from build123d import *

# Parameters (mm, degrees)
F0_W             = 20
F0_H             = 20
F1_DEPTH         = 448
F2_R             = 2.1
F3_DEPTH         = 448.001
F4_R             = 1
F6_DEPTH         = 448.001
F6_COPIES3_COUNT = 2
F6_COPIES3_ANGLE = 90
F6_COPIES4_COUNT = 2
F6_COPIES4_ANGLE = 270
F6_COPIES6_COUNT = 2
F9_W             = 16.4
F9_H             = 6.8613203436
F10_DEPTH        = 448.001
F12_DEPTH        = 448


# Not quite as in the source:
# - a pattern or mirror of a feature is missing from the dataset's text; its kind, count and spacing are read off the source's solid


with BuildPart() as f1:
    # F0 (on Front) → F1 (new body)
    with BuildSketch(Plane.XZ):
        Rectangle(F0_W, F0_H)
    extrude(amount=F1_DEPTH)

    # F2 (on face) → F3 (cut, through all)
    with BuildSketch(Plane.XZ.offset(448)):
        Circle(F2_R)
    extrude(amount=-F3_DEPTH, mode=Mode.SUBTRACT)

    # F4
    f4_edges = [f1.edges().sort_by_distance(p)[0] for p in [
        (-10, -224, 10),
        (10, -224, 10),
    ]]
    fillet(f4_edges, radius=F4_R)

    # F5 (on face) → F6 (cut, through all)
    with BuildSketch(Plane.XZ.offset(448)):
        Polygon((0, 3.9006601718), (0, 10), (-2.84, 10), (-4.64, 10), (-2.84, 8.2), (-5.4993398282, 8.2), (-5.4993398282, 6.56), (-2.84, 3.9006601718), align=None)
        Polygon((-6.5693398282, 8.2), (-8.2, 8.2), (-7.0953059148, 7.0953059148), (-6.5693398282, 7.6212720014), align=None)
    f6 = extrude(amount=-F6_DEPTH, mode=Mode.SUBTRACT)

    # F6_copies: F6 across plane
    add(f6.mirror(Plane(origin=(0, 0, 0), x_dir=(-0.7071067812, 0, -0.7071067812), z_dir=(0.7071067812, 0, -0.7071067812))), mode=Mode.SUBTRACT)

    # F6_copies1: F6 across plane
    add(f6.mirror(Plane(origin=(0, 0, 0), x_dir=(0.7071067812, 0, -0.7071067812), z_dir=(-0.7071067812, 0, -0.7071067812))), mode=Mode.SUBTRACT)

    # F6_copies2: F6 across plane
    add(f6.mirror(Plane(origin=(0, 0, 0), x_dir=(0, 0, 1), z_dir=(1, 0, 0))), mode=Mode.SUBTRACT)

    # F6_copies3: F6 ×2 about axis
    f6_copies3_axis = Axis((0, 0, 0), (0, 1, 0))
    for i in range(1, F6_COPIES3_COUNT):
        add(f6.rotate(f6_copies3_axis, i * F6_COPIES3_ANGLE / (F6_COPIES3_COUNT - 1)), mode=Mode.SUBTRACT)

    # F6_copies4: F6 ×2 about axis
    f6_copies4_axis = Axis((0, 0, 0), (0, 1, 0))
    for i in range(1, F6_COPIES4_COUNT):
        add(f6.rotate(f6_copies4_axis, i * F6_COPIES4_ANGLE / (F6_COPIES4_COUNT - 1)), mode=Mode.SUBTRACT)

    # F6_copies5: F6 across plane
    add(f6.mirror(Plane(origin=(0, 0, 0), x_dir=(-1, 0, 0), z_dir=(0, 0, -1))), mode=Mode.SUBTRACT)

    # F6_copies6: F6 ×2 about axis
    f6_copies6_axis = Axis((0, 0, 0), (0, 1, 0))
    for i in range(1, F6_COPIES6_COUNT):
        add(f6.rotate(f6_copies6_axis, i * 360 / F6_COPIES6_COUNT), mode=Mode.SUBTRACT)

    # F8: F1 across face


with BuildPart() as f1_1:
    add(f1.part)
    add(f1.part.mirror(Plane(origin=(-7.32, -224, -10), x_dir=(1, 0, 0), z_dir=(0, 0, -1))))

    # F9 (on face) → F10 (cut, through all)
    with BuildSketch(Plane.XZ.offset(448)):
        with Locations((0, -10)):
            Rectangle(F9_W, F9_H)
    extrude(amount=-F10_DEPTH, mode=Mode.SUBTRACT)

    # F11 (on face) → F12 (join, through all)
    with BuildSketch(Plane.XZ.offset(448)):
        with BuildLine():
            ThreePointArc((-9, -10), (-9.7071067812, -9.7071067812), (-10, -9))
            Line((-10, -9), (-10, -11))
            ThreePointArc((-10, -11), (-9.7071067812, -10.2928932188), (-9, -10))
        make_face()
        with BuildLine():
            ThreePointArc((10, -9), (9.7071067812, -9.7071067812), (9, -10))
            ThreePointArc((9, -10), (9.7071067812, -10.2928932188), (10, -11))
            Line((10, -11), (10, -9))
        make_face()
        Polygon((5.9386796564, -6.9993398282), (8.2, -6.9993398282), (8.2, -6.5693398282), (5.5086796564, -6.5693398282), align=None)
        Polygon((-8.2, -6.5693398282), (-8.2, -6.9993398282), (-5.9386796564, -6.9993398282), (-5.5086796564, -6.5693398282), align=None)
    extrude(amount=-F12_DEPTH)


solid = f1_1.part
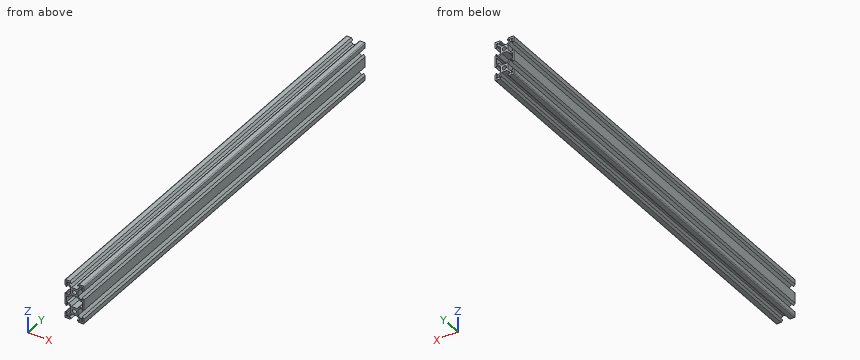
The model under review builds one solid part; all positions refer to its coordinate system, in mm. Give positions to 0.01 mm unless a question says otherwise; leave off trailing zeros. One line per question, with ' | ' between items. Start each with the question number.
Item 1: Wall thickness on line 1 (Z direction, x = 0, y = -333.5); line 2 (Z direction, x = 8, y = -54.5); line 3 (X direction, y = -407.5, z = 7): over which ranges is each line inside the solid? List them lowest first. Write a range as from..to.
Item 2: For pin 1 (3 mm diameter, centred on x = -4.5, y = -162, fed in from -Z); pin 2 (4 mm diameter, centred on y = -292, z = -22.5, fed in from +X); pin 3 (1.5 mm diameter, centred on y = -399.5, z = 3.5, fed in from +X); pin 4 (4.5 mm diameter, centred on x = -1, y = -185, fed in from +Z), all flat-tipped, find the tip position at first contact; note any pin that passes through.
Item 3: We need section A-A on y = -33. Give the number of separate pieces and of enclosed holes in the cut face, plus the area to 3 significant figures.
Results found:
1) line 1: z = -23.9..-22.1, -17.9..-16.1, -3.9..-2.1, 2.1..3.9 | line 2: z = -30..-28.2, -26.57..-25.5, -14.5..-13.43, -7..-5.5, 5.5..6.57, 8.2..10 | line 3: x = -10..-8.2, -7.19..-5.5, 5.5..7.19, 8.2..10
2) pin 1: stops at z = -30 | pin 2: stops at x = 9.86 | pin 3: stops at x = 9.61 | pin 4: stops at z = 8.61
3) separate pieces: 1 | enclosed holes: 7 | area: 286 mm2
